Could you check a few things on this model? Use its own coordinates, in mm. Face numbers are marked on the shaded views. A direction names the side the tool comes from. Coordinates: 2 decimals unless noted, no trailing zeros. Loops run counter-clockwise (first coordinate to the right, second up) from the corner with the lowest first, then second, coordinate; pieces in that order, holes last.
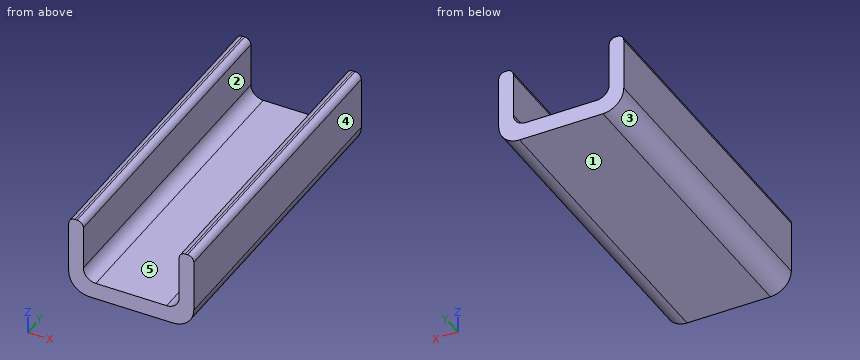
from build123d import *

# Parameters (mm, degrees)
F1_DEPTH = 15


with BuildPart() as f1:
    # F0 (on Front) → F1 (new body)
    with BuildSketch(Plane.XZ):
        with BuildLine():
            Line((-2.777976, 3.8), (-2.877976, 3.8))
            ThreePointArc((-2.877976, 3.8), (-3.090108, 3.712132), (-3.177976, 3.5))
            Line((-3.177976, 3.5), (-3.177976, 1))
            ThreePointArc((-3.177976, 1), (-2.885083, 0.292893), (-2.177976, 0))
            Line((-2.177976, 0), (1.822024, 0))
            ThreePointArc((1.822024, 0), (2.52913, 0.292893), (2.822024, 1))
            Line((2.822024, 1), (2.822024, 3.5))
            ThreePointArc((2.822024, 3.5), (2.734156, 3.712132), (2.522024, 3.8))
            Line((2.522024, 3.8), (2.422024, 3.8))
            ThreePointArc((2.422024, 3.8), (2.209892, 3.712132), (2.122024, 3.5))
            Line((2.122024, 3.5), (2.122024, 1.4))
            ThreePointArc((2.122024, 1.4), (1.946288, 0.975736), (1.522024, 0.8))
            Line((1.522024, 0.8), (-1.877976, 0.8))
            ThreePointArc((-1.877976, 0.8), (-2.30224, 0.975736), (-2.477976, 1.4))
            Line((-2.477976, 1.4), (-2.477976, 3.5))
            ThreePointArc((-2.477976, 3.5), (-2.565844, 3.712132), (-2.777976, 3.8))
        make_face()
    extrude(amount=-F1_DEPTH)


solid = f1.part
(1) Imagine slicing it at D-D, the plane z = 0.55. Write out the boundary of the cut face in (x, y), and give its area (3 significant figures).
Answers:
outline: (-3.07, 0) - (2.72, 0) - (2.72, 15) - (-3.07, 15) - close
area: 86.8 mm2
(2) Imagine slicing it at A-A, the plane z = 2.95. Write out the boundary of the cut face in (x, y), and give its area (3 significant figures).
Answers:
outline: (-3.18, 0) - (-2.48, 0) - (-2.48, 15) - (-3.18, 15) - close; (2.12, 0) - (2.82, 0) - (2.82, 15) - (2.12, 15) - close
area: 21.0 mm2
(3) I need wall thicknesses on probe 1 along X at (y, z) = (14.25, 1.4); probe 2 along Z at (x, y) = (0.75, 12); probe 3 along X at (y, z) = (10, 0.7). Which ranges of each line are inside material? Lowest first, please.
Answers:
probe 1: x = -3.18 to -2.48, 2.12 to 2.82
probe 2: z = 0 to 0.8
probe 3: x = -3.13 to 2.78
(4) We'd pull the mould along X, two halves only. Please class the marked faces 1, 2 and 3: +X half, -X half, draft (parallel to the pull), parting line (faces both ways), or undercut.
Answers:
face 1: draft
face 2: undercut
face 3: -X half
(5) For pin 1 (1.5 mm diameter, centred on x = -1.5, z = 1, fed in from -Y); pin 2 (1.7 mm diameter, centred on x = 0, y = 6.5, fed in from +Z), each with a flat end and sliding along its axis, tell me the tip position at first contact or that it passes through.
Answers:
pin 1: stops at y = 0
pin 2: stops at z = 0.8
(6) Imagine slicing it at C-C, the plane x = -1. Write out the boundary of the cut face in (y, z).
Answers:
outline: (0, 0) - (15, 0) - (15, 0.8) - (0, 0.8) - close
(7) Imagine slicing it at B-B, the plane y = 9.25. Write out the boundary of the cut face in (x, z).
Answers:
outline: (-3.18, 1) arc R1 ccw to (-2.18, 0) - (1.82, 0) arc R1 ccw to (2.82, 1) - (2.82, 3.5) arc R0.3 ccw to (2.52, 3.8) - (2.42, 3.8) arc R0.3 ccw to (2.12, 3.5) - (2.12, 1.4) arc R0.6 cw to (1.52, 0.8) - (-1.88, 0.8) arc R0.6 cw to (-2.48, 1.4) - (-2.48, 3.5) arc R0.3 ccw to (-2.78, 3.8) - (-2.88, 3.8) arc R0.3 ccw to (-3.18, 3.5) - close
(8) Which directions (+Z, -Z, +X, -X, +Y, -Y) give clear straight access to the entire face, cutting with the end or side of a thin tool? Please do the marked faces 4 and 5.
Answers:
face 4: +Z, -Z, +X, +Y, -Y
face 5: +Z, +Y, -Y
